```python
from build123d import *

# Parameters (mm, degrees)
SKETCH1_W                                      = 10
SKETCH1_H                                      = 10
FOOT_DEPTH                                     = 5
SKETCH2_W                                      = 10
SKETCH2_H                                      = 8
LEG_DEPTH                                      = 14
SKETCH3_R                                      = 5
HIP_CONNECTOR_DEPTH                            = 10
SKETCH20_R                                     = 3.5
DECORATIVE_CIRCLE_THAT_MAKES_THIS_EASY_T_DEPTH = 0.1
HIP_ROOM_DEPTH                                 = 1.5
HIP_HOLE_D                                     = 4
HIP_HOLE_DEPTH                                 = 6
HIP_HOLE_TIP                                   = 1.201721238
SKETCH18_W                                     = 6
SKETCH18_H                                     = 6
FOOT_HOLE_DEPTH                                = 2.5
WEIGHT_REDUCTION_MAKE_IT_EASY_TO_ADD_CEN_D     = 3
WEIGHT_REDUCTION_MAKE_IT_EASY_TO_ADD_CEN_DEPTH = 8
WEIGHT_REDUCTION_MAKE_IT_EASY_TO_ADD_CEN_TIP   = 0.901290929
SKETCH19_W                                     = 10
SKETCH19_H                                     = 20
THIGH_GAP_DEPTH                                = 0.25
SCALE1_SCALE                                   = 2


with BuildPart() as part:
    # Sketch1 → Foot (new body)
    with BuildSketch(Plane(origin=(0, 0, 0), x_dir=(1, 0, 0), z_dir=(0, 1, 0))):
        with Locations((5, -5)):
            Rectangle(SKETCH1_W, SKETCH1_H)
    extrude(amount=FOOT_DEPTH)

    # Sketch2 → Leg (add)
    with BuildSketch(Plane(origin=(0, 5, 0), x_dir=(1, 0, 0), z_dir=(0, 1, 0))):
        with Locations((5, -4)):
            Rectangle(SKETCH2_W, SKETCH2_H)
    extrude(amount=LEG_DEPTH)

    # Sketch3 → Hip Connector (add)
    with BuildSketch(Plane(origin=(0, 0, 0), x_dir=(0, 0, -1), z_dir=(1, 0, 0))):
        with Locations((-5, 19)):
            Circle(SKETCH3_R)
    extrude(amount=HIP_CONNECTOR_DEPTH)

    # Sketch20 → Decorative circle that makes this easy to dimension (cut)
    with BuildSketch(Plane.ZY):
        with Locations((5, 19)):
            Circle(SKETCH20_R)
    extrude(amount=-DECORATIVE_CIRCLE_THAT_MAKES_THIS_EASY_T_DEPTH, mode=Mode.SUBTRACT)

    # Sketch4 → Hip room (cut)
    with BuildSketch(Plane(origin=(10, 0, 0), x_dir=(0, 0, -1), z_dir=(1, 0, 0))):
        with BuildLine():
            Line((-5, 13.99), (-10, 13.99))
            Line((-10, 13.99), (-10, 24))
            Line((-10, 24), (0, 24))
            Line((0, 24), (0, 16.101701649))
            Line((0, 16.101701649), (-2.495, 14.661212727))
            ThreePointArc((-2.495, 14.661212727), (-3.703316584, 14.16071161), (-5, 13.99))
        make_face()
    extrude(amount=-HIP_ROOM_DEPTH, mode=Mode.SUBTRACT)

    # Hip hole
    with Locations(Plane(origin=(8.5, 0, 0), x_dir=(0, 0, -1), z_dir=(1, 0, 0))):
        with Locations((-5, 19)):
            Hole(HIP_HOLE_D / 2, depth=HIP_HOLE_DEPTH)
            with Locations((0, 0, -(HIP_HOLE_DEPTH + HIP_HOLE_TIP / 2))):  # 118° drill point
                Cone(0, HIP_HOLE_D / 2, HIP_HOLE_TIP, mode=Mode.SUBTRACT)

    # Sketch18 → Foot hole (cut)
    with BuildSketch(Plane.XZ):
        with Locations((5, 5)):
            Rectangle(SKETCH18_W, SKETCH18_H)
    extrude(amount=-FOOT_HOLE_DEPTH, mode=Mode.SUBTRACT)

    # Weight reduction/make it easy to add centerline hole
    with Locations(Plane(origin=(0, 2.5, 0), x_dir=(-1, 0, 0), z_dir=(0, -1, 0))):
        with Locations((-5, -5)):
            Hole(WEIGHT_REDUCTION_MAKE_IT_EASY_TO_ADD_CEN_D / 2, depth=WEIGHT_REDUCTION_MAKE_IT_EASY_TO_ADD_CEN_DEPTH)
            with Locations((0, 0, -(WEIGHT_REDUCTION_MAKE_IT_EASY_TO_ADD_CEN_DEPTH + WEIGHT_REDUCTION_MAKE_IT_EASY_TO_ADD_CEN_TIP / 2))):  # 118° drill point
                Cone(0, WEIGHT_REDUCTION_MAKE_IT_EASY_TO_ADD_CEN_D / 2, WEIGHT_REDUCTION_MAKE_IT_EASY_TO_ADD_CEN_TIP, mode=Mode.SUBTRACT)

    # Sketch19 → Thigh gap (cut)
    with BuildSketch(Plane(origin=(10, 0, 0), x_dir=(0, 0, -1), z_dir=(1, 0, 0))):
        with Locations((-5, 10)):
            Rectangle(SKETCH19_W, SKETCH19_H)
    extrude(amount=-THIGH_GAP_DEPTH, mode=Mode.SUBTRACT)


with BuildPart() as part_1:
    # Scale1: scaled about (4.599513464, 11.496150449, 4.477610723)
    add(part.part.scale(SCALE1_SCALE).moved(Location((-4.599513464, -11.496150449, -4.477610723))))


solid = part_1.part
```
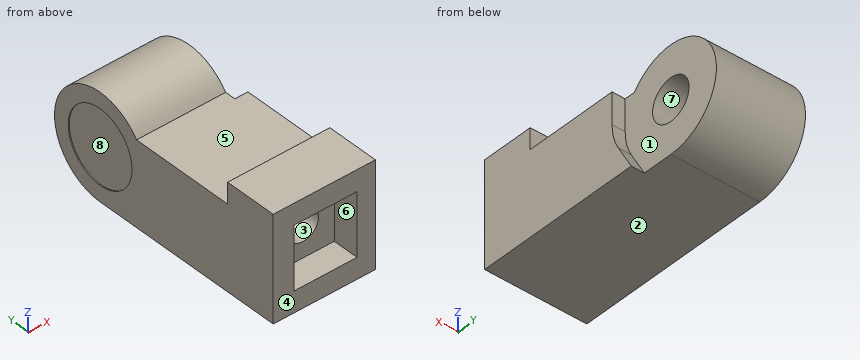
Build history of the part. All positions in model axes, mm. Face numbers are marked on the shaded views. A direction names the side the tool comes from. Round coordinates to 2 decimals unless told otherwise and drop trailing zeros. Write each loop counter-clockwise with the first axis right and the second up, starting at its lowest first coordinate (ties: lowest second). Pieces come first, ordered by that corner, then holes. Notation, with made-up numbers: (35, 25) -> (63, 25) arc R24 cw to (63, 61) -> close; hole circle Ø8 at (-39.5, -1.5). An arc over 180 degrees is marked (long way). Put each result on its own line as item: value.
Item 1: Slice it at A-A, the plane x = 9.5. Give the cut face in (y, z), plus the area to 3 significant figures.
Here are the results:
outline: (-11.5, -4.48) -> (26.5, -4.48) arc R10 ccw (long way) to (18.5, 11.52) -> (-1.5, 11.52) -> (-1.5, 15.52) -> (-11.5, 15.52) -> (-11.5, 11.52) -> (-6.5, 11.52) -> (-6.5, -0.48) -> (-11.5, -0.48) -> close; hole circle Ø8 at (26.5, 5.52)
area: 717 mm^2
Item 2: Slice it at D-D, the plane y = 16. Give the cut face in (x, z), plus the area to 3 significant figures.
Here are the results:
outline: (-4.6, -4.48) -> (14.9, -4.48) -> (14.9, 11.52) -> (-4.6, 11.52) -> close
area: 312 mm^2
Item 3: Slice it at C-C, the plane x = 13. Give the cut face in (y, z).
Here are the results:
outline: (-11.5, -4.48) -> (20.71, -4.48) -> (17.83, 0.51) arc R10.02 cw to (16.48, 5.52) -> (16.48, 11.52) -> (-1.5, 11.52) -> (-1.5, 15.52) -> (-11.5, 15.52) -> close
Item 4: Two-plate mould, pull along X, no slides. Class the marked faces 1, 2 and 3: pulls with the +X half, pulls with the -X half, needs draft (parallel to the pull), parting line crosses it, or undercut.
Here are the results:
face 1: pulls with the +X half
face 2: needs draft
face 3: undercut
Item 5: Flat gauge pins, fed straight in: P1, Ø1.2, axis at x = 1.5, z = 14, coming from the +Y side; P2, Ø0.8, axis at x = 13.5, z = 8.5, coming from the +Y side; P3, Ø5, axis at x = 5.4, z = 5.52, coming from the -Y side. Where does each tip first touch, or does it go through?
Here are the results:
P1: stops at y = 32.66
P2: stops at y = 16.48
P3: stops at y = 9.8
Item 6: Wall check: probe 1 along Y at (x, z) = (10, 5.25); probe 2 along Z at (x, y) = (6.25, 6.5); probe 3 along Z at (x, y) = (9.5, 23.5). Give the ranges that are in metal, low to high. Write a range as from..to.
Here are the results:
probe 1: y = -6.5..22.51, 30.49..36.5
probe 2: z = -4.48..2.65, 8.4..11.52
probe 3: z = -4.48..2.88, 8.16..15.06
Item 7: Slice it at B-B, the plane z = 13.75. Give the cut face in (x, y), plus the area to 3 significant figures.
Here are the results:
outline: (-4.6, -11.5) -> (14.9, -11.5) -> (14.9, -1.5) -> (-4.6, -1.5) -> close; (-4.6, 20.82) -> (12.4, 20.82) -> (12.4, 32.19) -> (-4.6, 32.19) -> close
area: 388 mm^2
Item 8: Tool access for the marked faces 4, 5, 6, 7 and 8: list every direction of +Z, -Z, +X, -X, +Y, -Y with a clear straight run to the whole face (end or side of a thin tool).
Here are the results:
face 4: +Z, -Z, +X, -X, -Y
face 5: +Z, +X, -X
face 6: -Y
face 7: +X
face 8: -X
